Read the model definition and answer for the solid it produces. Units are mm, in the model's axes. Round coordinates to 2 decimals unless told otherwise and drop trailing zeros.
from build123d import *

# Parameters (mm, degrees)
SKETCH1_R           = 2.5
BOSS_EXTRUDE1_DEPTH = 120
FILLET1_R           = 1
FILLET2_R           = 0.5
FILLET3_R           = 0.5
FILLET4_R           = 0.5
FILLET5_R           = 0.5
SKETCH2_R           = 2.5
CUT_EXTRUDE1_DEPTH  = 8


with BuildPart() as part:
    # Sketch1 → Boss-Extrude1 (new body)
    with BuildSketch(Plane.XY):
        Polygon((13.2, 0), (13.2, 1.8), (15.45, 1.8), (15.45, 3.6), (12.95, 6.1), (7.05, 6.1), (4.55, 3.6), (4.55, 1.8), (6.8, 1.8), (6.8, 0), (0, 0), (0, 6.8), (1.8, 6.8), (1.8, 4.55), (3.6, 4.55), (6.1, 7.05), (6.1, 12.95), (3.6, 15.45), (1.8, 15.45), (1.8, 13.2), (0, 13.2), (0, 20), (6.8, 20), (6.8, 18.2), (4.55, 18.2), (4.55, 16.4), (7.05, 13.9), (12.95, 13.9), (15.45, 16.4), (15.45, 18.2), (13.2, 18.2), (13.2, 20), (20, 20), (20, 13.2), (18.2, 13.2), (18.2, 15.45), (16.4, 15.45), (13.9, 12.95), (13.9, 7.05), (16.4, 4.55), (18.2, 4.55), (18.2, 6.8), (20, 6.8), (20, 0), align=None)
        with Locations((10, 10)):
            Circle(SKETCH1_R, mode=Mode.SUBTRACT)
    extrude(amount=BOSS_EXTRUDE1_DEPTH)

    # Fillet1
    fillet1_edges = [part.edges().sort_by_distance(p)[0] for p in [
        (0, 0, 60),
        (0, 20, 60),
        (20, 20, 60),
        (20, 0, 60),
    ]]
    fillet(fillet1_edges, radius=FILLET1_R)

    # Fillet2
    fillet2_edges = [part.edges().sort_by_distance(p)[0] for p in [
        (4.55, 18.2, 60),
        (4.55, 16.4, 60),
        (7.05, 13.9, 60),
        (12.95, 13.9, 60),
        (15.45, 16.4, 60),
        (15.45, 18.2, 60),
    ]]
    fillet(fillet2_edges, radius=FILLET2_R)

    # Fillet3
    fillet3_edges = [part.edges().sort_by_distance(p)[0] for p in [
        (18.2, 15.45, 60),
        (16.4, 15.45, 60),
        (13.9, 12.95, 60),
        (13.9, 7.05, 60),
        (16.4, 4.55, 60),
        (18.2, 4.55, 60),
    ]]
    fillet(fillet3_edges, radius=FILLET3_R)

    # Fillet4
    fillet4_edges = [part.edges().sort_by_distance(p)[0] for p in [
        (1.8, 4.55, 60),
        (3.6, 4.55, 60),
        (6.1, 7.05, 60),
        (6.1, 12.95, 60),
        (3.6, 15.45, 60),
        (1.8, 15.45, 60),
    ]]
    fillet(fillet4_edges, radius=FILLET4_R)

    # Fillet5
    fillet5_edges = [part.edges().sort_by_distance(p)[0] for p in [
        (15.45, 1.8, 60),
        (15.45, 3.6, 60),
        (12.95, 6.1, 60),
        (7.05, 6.1, 60),
        (4.55, 3.6, 60),
        (4.55, 1.8, 60),
    ]]
    fillet(fillet5_edges, radius=FILLET5_R)

    # Sketch2 → Cut-Extrude1 (cut)
    with BuildSketch(Plane(origin=(0, 13.9, 0), x_dir=(1, 0, 0), z_dir=(0, 1, 0))):
        with Locations((10, -60)):
            Circle(SKETCH2_R)
        with Locations((10, -80)):
            Circle(SKETCH2_R)
        with Locations((10, -40)):
            Circle(SKETCH2_R)
    extrude(amount=-CUT_EXTRUDE1_DEPTH, mode=Mode.SUBTRACT)


solid = part.part
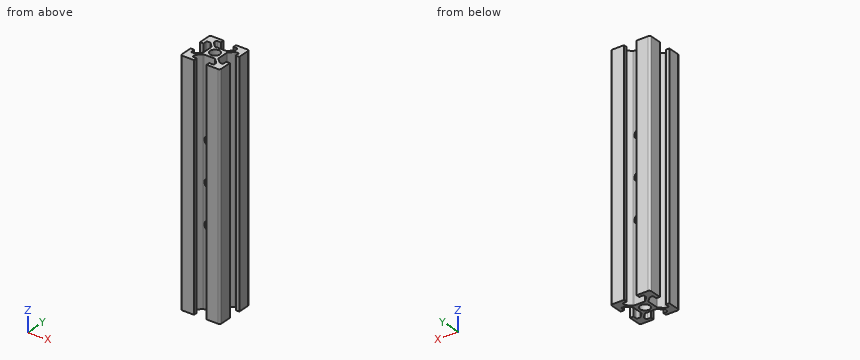
Q1. A cutting plane is placed at A-A, the plane x = 10. Give the number of separate pieces and of enclosed holes in the cut face, plus the area to 3 significant figures.
Outcome:
separate pieces: 8
enclosed holes: 0
area: 294 mm2
Q2. Flat-ended cylindrical pins translate along their axes: pin 1 (5 mm diameter, centred on x = 10, z = 107, fed in from +Y); pin 2 (6 mm diameter, centred on x = 10, z = 42.5, fed in from -Y); pin 3 (4 mm diameter, centred on y = 9, z = 13.5, fed in from +X). Find the tip coordinate at first contact, or state that the pin passes through.
Outcome:
pin 1: stops at y = 13.9
pin 2: stops at y = 6.03
pin 3: stops at x = 13.97
Q3. Straight lines are drawn through the part: probe 1 along X at (y, z) = (1, 96.5); probe 2 along Y at (x, z) = (3.25, 80.5). For each, find the intervals that lie inside material, in ascending order.
Outcome:
probe 1: x = 0 to 6.8, 13.2 to 20
probe 2: y = 0 to 4.55, 15.45 to 20
